Geometry check sheet. Reference: the model listing, model coordinates, mm. A direction names the side the tool comes from. Coordinates: 2 decimals unless noted, no trailing zeros. Write each loop counter-clockwise with the first axis right and the second up, starting at its lowest first coordinate (ties: lowest second). Pieces come first, ordered by that corner, then holes. Notation, with made-up numbers: (58, 14.25) -> (88, 14.25) arc R34 ccw to (88, 51.25) -> close; hole circle Ø10 at (30.25, 42). An arc over 180 degrees is marked (long way). Answer in a Markdown table with one row per item. Add a question column.
Q1. Section check B-B, the plane y = 50. Record the boundary of the cut face in (x, z), and give its area (3 significant figures).
Q2. Tool access check on faces 4 (the face through (108, 4, 123)), 5 (the face through (109, 2, 0)). Record the directions out of +Z, -Z, +X, -X, +Y, -Y that give a thin tool (end or side, any length) a straight path to the whole face; none if there is none.
Q3. Release check for a two-part mould opening along Y. For faces 1 (the face through (111.58, 106.134, 123.25)), 2 (the face through (0, 39, 123)), 3 (the face through (108, 0, 123)) record: pulls with the +Y half, pulls with the -Y half, needs draft (parallel to the pull), parting line crosses it, or undercut.
Q4. Gauge pin test, flat ends, axial feed: P1, Ø6, axis at x = 63, z = 35, coming from the +Y side; P2, Ø8, axis at x = 172, z = 71, coming from the +Y side. Record the tip position at first contact, or that the pin passes through.
Q5. Section check C-C, the plane x = 74. Record the boundary of the cut face in (y, z), and give its area (3 significant figures).
Q6. Thickness scan on line 1 (X direction, y = 44.5, z = 17); line 2 (Y direction, x = 26, z = 237.5); line 3 (Y direction, x = 78, z = 230). Record the ranges inside material, lowest first.
Q7. Section check A-A, the plane z = 183. Record the boundary of the cut face in (x, y), and give its area (3 significant figures).
```python
from build123d import *

# Parameters (mm, degrees)
PAD_DEPTH = 250


with BuildPart() as part:
    # Sketch → Pad (new body)
    with BuildSketch(Plane.XY):
        with BuildLine():
            Line((0, 0), (220, 0))
            Line((220, 0), (220, 80))
            ThreePointArc((220, 80), (110, 108.140114), (0, 80))
            Line((0, 0), (0, 80))
        make_face()
        with BuildLine():
            Line((2, 4), (218, 4))
            Line((218, 4), (218, 78))
            ThreePointArc((218, 78), (110, 106.140114), (2, 78))
            Line((2, 4), (2, 78))
        make_face(mode=Mode.SUBTRACT)
    extrude(amount=PAD_DEPTH)


solid = part.part
```
Calculated:
| question | item | result |
|---|---|---|
| 1 | outline | (0, 0) -> (2, 0) -> (2, 250) -> (0, 250) -> close; (218, 0) -> (220, 0) -> (220, 250) -> (218, 250) -> close |
| 1 | area | 1,000 mm² |
| 2 | face 4 | +Z, -Z |
| 2 | face 5 | -Z, +X, -X, +Y, -Y |
| 3 | face 1 | undercut |
| 3 | face 2 | needs draft |
| 3 | face 3 | pulls with the -Y half |
| 4 | P1 | stops at y = 103.87 |
| 4 | P2 | stops at y = 100.68 |
| 5 | outline | (0, 0) -> (4, 0) -> (4, 250) -> (0, 250) -> close; (103.19, 0) -> (105.29, 0) -> (105.29, 250) -> (103.19, 250) -> close |
| 5 | area | 1,530 mm² |
| 6 | line 1 | x = 0 to 2, 218 to 220 |
| 6 | line 2 | y = 0 to 4, 89.58 to 92.18 |
| 6 | line 3 | y = 0 to 4, 103.81 to 105.89 |
| 7 | outline | (0, 0) -> (220, 0) -> (220, 80) arc R229.07 ccw to (0, 80) -> close; hole (2, 4) -> (218, 4) -> (218, 78) arc R221.32 ccw to (2, 78) -> close |
| 7 | area | 1,690 mm² |
